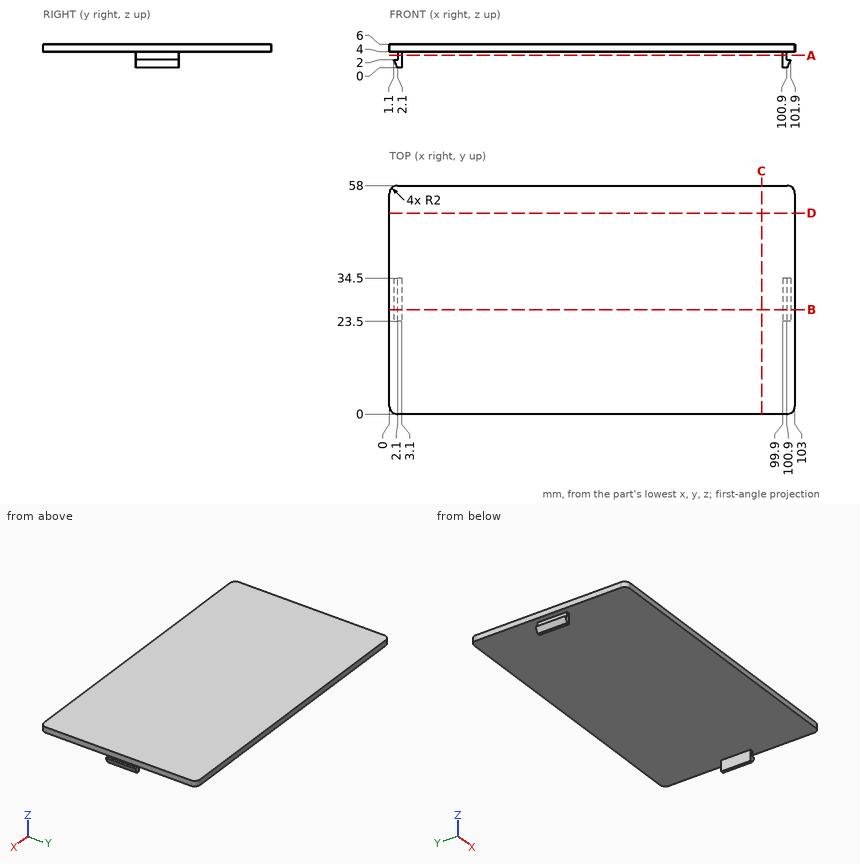
Geometry check sheet. Reference: drawing and pictorial views, mm from the part's lowest x, y, z. Give positions to 0.01 mm unless a question says otherwise; leave off trailing zeros. Write each loop counter-clockwise with the first axis right and the second up, starting at its lowest first coordinate (ties: lowest second). Pieces come first, ordered by that corner, then holes. Notation, with made-up numbers: M -32,-39.75 L 6,-39.75 A25 ccw 6,-7.75 Z; hole C 80.5,32 d5. An arc over 180 degrees is marked long. Use CSV: the item, a comma, the result in double quotes.
1) Material ranges on line 1 along X through (y, z) = (33, 2.7); line 2 along Z through (x, y) = (69, 27); line 3 along X through (y, z) = (31, 0.55) (3 decimals), recorded low to high.
Final values:
line 1,"2.1 to 3.1, 99.9 to 100.9"
line 2,"4 to 6"
line 3,"1.825 to 3.1, 99.9 to 101.175"
2) Cross-section at D-D (y = 51). Enter the section's corners in (x, z), plus the area to 3 significant figures.
Final values:
outline,"M 0,4 L 103,4 L 103,6 L 0,6 Z"
area,"206 mm²"
3) Cross-section at C-C (x = 94.5). Enter the section's corners in (y, z), plus the area to 3 significant figures.
Final values:
outline,"M 0,4 L 58,4 L 58,6 L 0,6 Z"
area,"116 mm²"
4) Go/stop test with flat-tipped pins: pin 1 Ø1.5 at (y, z) = (28, 2.5) entering from -X; pin 2 Ø2 at (x, z) = (101.5, 1) entering from -Y; pin 3 Ø8 at (x, y) = (66.5, 35) entering from -Z. Record where each tip stops, or that it passes through.
Final values:
pin 1,"x = 1.1"
pin 2,"y = 23.5"
pin 3,"z = 4"
5) Cross-section at A-A (z = 3.1). Enter the section's corners in (x, y), plus the area to 3 significant figures.
Final values:
outline,"M 2.1,23.5 L 3.1,23.5 L 3.1,34.5 L 2.1,34.5 Z; M 99.9,23.5 L 100.9,23.5 L 100.9,34.5 L 99.9,34.5 Z"
area,"22.0 mm²"
6) Cross-section at B-B (y = 26.5). Enter the section's corners in (x, z).
Final values:
outline,"M 0,4 L 2.1,4 L 2.1,2 L 1.1,2 L 2.1,0 L 3.1,0 L 3.1,4 L 99.9,4 L 99.9,0 L 100.9,0 L 101.9,2 L 100.9,2 L 100.9,4 L 103,4 L 103,6 L 0,6 Z"
